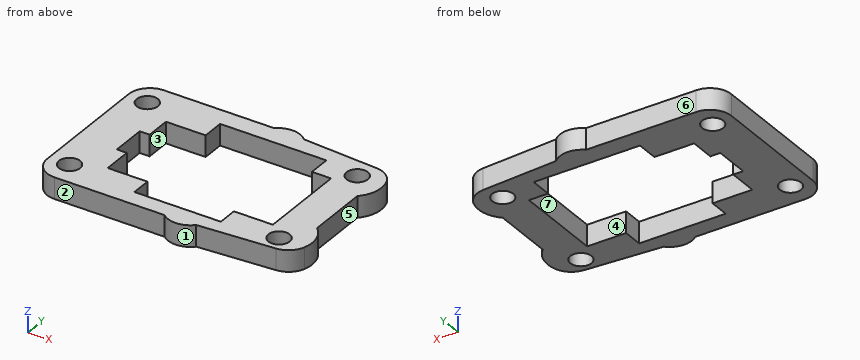
from build123d import *

# Parameters (mm, degrees)
ESQUISSE1_R               = 1.5
T_LE_DE_BASE_PLI_E1_DEPTH = 3


# Sheet-metal steps are written as plain solids
with BuildPart() as part:
    # Esquisse1 → Tôle de base pliée1 (new body)
    with BuildSketch(Plane.XY):
        with BuildLine():
            Line((1210.954881098, 2192.062900441), (1210.954881098, 2174.562900441))
            ThreePointArc((1210.954881098, 2174.562900441), (1211.833560754, 2172.441580098), (1213.954881098, 2171.562900441))
            Line((1213.954881098, 2171.562900441), (1229.498862267, 2171.562900441))
            ThreePointArc((1229.498862267, 2171.562900441), (1231.700410864, 2170.796575468), (1233.830537909, 2171.743480404))
            Line((1233.830537909, 2171.743480404), (1244.602630734, 2172.48006345))
            ThreePointArc((1244.602630734, 2172.48006345), (1246.258569693, 2173.112570346), (1247.278053022, 2174.56269191))
            ThreePointArc((1247.278053022, 2174.56269191), (1247.351627268, 2176.949418696), (1246.12416641, 2178.997641771))
            Line((1246.12416641, 2178.997641771), (1246.12416641, 2187.628159112))
            ThreePointArc((1246.12416641, 2187.628159112), (1247.351627268, 2189.676382187), (1247.278053022, 2192.063108973))
            ThreePointArc((1247.278053022, 2192.063108973), (1246.258569693, 2193.513230537), (1244.602630734, 2194.145737433))
            Line((1244.602630734, 2194.145737433), (1233.830537909, 2194.882320479))
            ThreePointArc((1233.830537909, 2194.882320479), (1231.700410864, 2195.829225415), (1229.498862267, 2195.062900441))
            Line((1229.498862267, 2195.062900441), (1213.954881098, 2195.062900441))
            ThreePointArc((1213.954881098, 2195.062900441), (1211.833560754, 2194.184220785), (1210.954881098, 2192.062900441))
        make_face()
        with Locations((1243.604881098, 2191.458119207)):
            Circle(ESQUISSE1_R, mode=Mode.SUBTRACT)
        with Locations((1213.854881098, 2191.662900441)):
            Circle(ESQUISSE1_R, mode=Mode.SUBTRACT)
        with Locations((1213.854881098, 2174.962900441)):
            Circle(ESQUISSE1_R, mode=Mode.SUBTRACT)
        with Locations((1243.604881098, 2174.670527055)):
            Circle(ESQUISSE1_R, mode=Mode.SUBTRACT)
        Polygon((1241.354881098, 2189.262900441), (1241.354881098, 2176.762900441), (1235.854881098, 2176.762900441), (1235.854881098, 2173.962900441), (1223.654881098, 2173.962900441), (1223.654881098, 2176.762900441), (1218.054881098, 2176.762900441), (1218.054881098, 2180.862900441), (1216.654881098, 2180.862900441), (1216.654881098, 2185.762900441), (1218.054881098, 2185.762900441), (1218.054881098, 2189.262900441), (1223.654881098, 2189.262900441), (1223.654881098, 2192.362900441), (1238.654881098, 2192.362900441), (1238.654881098, 2189.262900441), align=None, mode=Mode.SUBTRACT)
    extrude(amount=-T_LE_DE_BASE_PLI_E1_DEPTH)


solid = part.part
For this review, take the finished solid that the model builds, in its own axes (mm). Face numbers are marked on the shaded views. A direction names the side the tool comes from. Round coordinates to 2 decimals unless told otherwise and drop trailing zeros. Order: outer loops, then holes, each group sorted by start corner. A loop starts at its lowest first (then second) coordinate and runs counter-clockwise, first axis right, second up. Notation, with made-up numbers: M 48.25,23 L 62.25,23 A27 ccw 62.25,62 Z; hole C 46.5,-14 d11. An arc over 180 degrees is marked long. Use a Markdown table: item, result. Add a question column.
Item 1: Tool access review of the marked faces 5, 6 and 7: name each direction out of +Z, -Z, +X, -X, +Y, -Y from which nothing blocks a thin tool from reaching the whole face with its end or side.
Item 2: Insertion check: pin 1 (1.5 mm diameter, centred on x = 1237.5, z = -2, fed in from -Y); pin 2 (0.7 mm diameter, centred on x = 1217, z = -2, fed in from -Y); pin 3 (0.9 mm diameter, centred on x = 1228, z = -1, fed in from +Y); pin 4 (2.5 mm diameter, centred on x = 1243.6, y = 2191.46, fed in from -Z) (3 decimals). Each pin has a flat end and moves straight along its axis. Give the tip position at first contact, or say it passes through.
Item 3: Add section A-A, the plane y = 2179.5. Give the boundary of the cut face in (x, z), then the cut area to 3 significant figures.
Item 4: Add section C-C, the plane y = 2175.75. Give the boundary of the cut face in (x, z), then the cut area to 3 significant figures.
Item 5: Add section B-B, the plane x = 1240.5. Give the boundary of the cut face in (y, z), then the cut area to 3 significant figures.
Item 6: Add section D-D, the plane z = -2.15. State how many separate pieces and enclosed holes the cut face has, then the cut area to 3 significant figures.
Item 7: Mouldability with a two-part tool opening along X and no side actions: class the marked faces 1, 2, 3 and 4 as released by +X, released by -X, zero draft, split by the parting line, or undercut.
Item 8: To check wall thickness, follow line 1 along X through (y, z) = (2186.5, -0.5); line 2 along X through (y, z) = (2184.5, -2); line 3 along Y through (x, z) = (1220, -0.35). State the ranges of each line that lie inside material, in increasing order.
Geometry results:
| question | item | result |
|---|---|---|
| 1 | face 5 | +Z, -Z, +X |
| 1 | face 6 | +Z, -Z, -X, +Y |
| 1 | face 7 | +Z, -Z |
| 2 | pin 1 | stops at y = 2171.94 |
| 2 | pin 2 | stops at y = 2171.56 |
| 2 | pin 3 | stops at y = 2195.06 |
| 2 | pin 4 | passes through |
| 3 | outline | M 1210.95,-3 L 1218.05,-3 L 1218.05,0 L 1210.95,0 Z; M 1241.35,-3 L 1246.12,-3 L 1246.12,0 L 1241.35,0 Z |
| 3 | area | 35.6 mm² |
| 4 | outline | M 1210.95,-3 L 1212.58,-3 L 1212.58,0 L 1210.95,0 Z; M 1215.13,-3 L 1223.65,-3 L 1223.65,0 L 1215.13,0 Z; M 1235.85,-3 L 1242.56,-3 L 1242.56,0 L 1235.85,0 Z; M 1244.65,-3 L 1247.49,-3 L 1247.49,0 L 1244.65,0 Z |
| 4 | area | 59.1 mm² |
| 5 | outline | M 2172.2,-3 L 2176.76,-3 L 2176.76,0 L 2172.2,0 Z; M 2189.26,-3 L 2194.43,-3 L 2194.43,0 L 2189.26,0 Z |
| 5 | area | 29.2 mm² |
| 6 | separate pieces | 1 |
| 6 | enclosed holes | 5 |
| 6 | area | 416 mm² |
| 7 | face 1 | split by the parting line |
| 7 | face 2 | zero draft |
| 7 | face 3 | undercut |
| 7 | face 4 | undercut |
| 8 | line 1 | x = 1210.95 to 1218.05, 1241.35 to 1246.12 |
| 8 | line 2 | x = 1210.95 to 1216.65, 1241.35 to 1246.12 |
| 8 | line 3 | y = 2171.56 to 2176.76, 2189.26 to 2195.06 |
